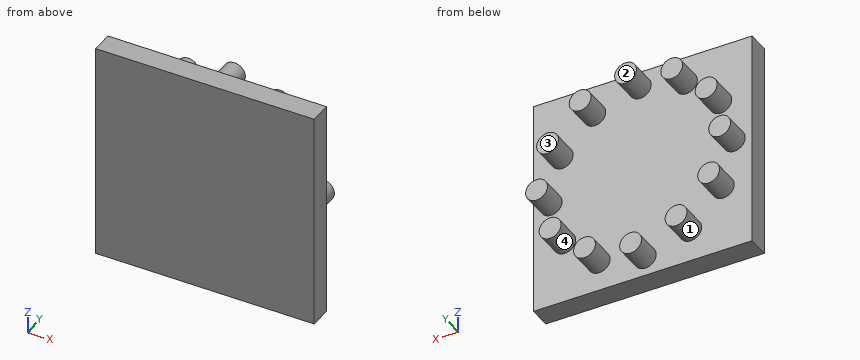
```python
from build123d import *

# Parameters (mm, degrees)
CROQUIS1_W              = 100
CROQUIS1_H              = 100
SALIENTE_EXTRUIR1_DEPTH = 10
CROQUIS2_R              = 5
SALIENTE_EXTRUIR2_DEPTH = 12
MATRIZC1_COUNT          = 12


with BuildPart() as part:
    # Croquis1 → Saliente-Extruir1 (new body)
    with BuildSketch(Plane(origin=(0, 0, 0), x_dir=(1, 0, 0), z_dir=(0, 1, 0))):
        Rectangle(CROQUIS1_W, CROQUIS1_H)
    extrude(amount=SALIENTE_EXTRUIR1_DEPTH)

    # Croquis2 → Saliente-Extruir2 (add)
    with BuildSketch(Plane(origin=(0, 10, 0), x_dir=(1, 0, 0), z_dir=(0, 1, 0))):
        with Locations(Location((-1.140405964, 41.553542307, 0), (0, 0, 270))):
            Circle(CROQUIS2_R)
    saliente_extruir2 = extrude(amount=SALIENTE_EXTRUIR2_DEPTH)

    # MatrizC1: Saliente-Extruir2 ×12 about axis
    matrizc1_axis = Axis((0.00902763, 0, 0.32894428), (0, 1, 0))
    for i in range(1, MATRIZC1_COUNT):
        add(saliente_extruir2.rotate(matrizc1_axis, i * 360 / MATRIZC1_COUNT))


solid = part.part
```
Check sheet for the modelled part. Datum: model origin and axes. Units: mm. Face numbers are marked on the shaded views. A direction names the side the tool comes from. Give positions to 0.01 mm unless a question says otherwise; leave off trailing zeros. Write each loop counter-clockwise with the first axis right and the second up, starting at its lowest first coordinate (ties: lowest second). Pieces come first, ordered by that corner, then holes. Notation, with made-up numbers: (0, 84.5) -> (8, 84.5) arc R21 cw to (8, 94.5) -> close; hole circle Ø1 at (19, 53). An arc over 180 degrees is marked (long way). Use CSV: the item, a comma, the result in double quotes. Start each with the question number.
Q1. Cross-section at D-D on x = -12.5. Enter the section's corners in (y, z), and give its area (3 significant figures).
Q2. Release check for a two-part mould opening along Z. For the marked faces 3 and 4 record: +Z half, -Z half, draft (parallel to the pull), parting line (faces both ways), or undercut.
Q3. Cross-section at A-A on y = 16. Count the separate pieces of the cut face and the enclosed holes in it, and give its area (3 significant figures).
Q4. Depth check by flat-ended pin: P1, Ø6, axis at x = -5, z = 21, coming from the +Y side. Enter the tip coordinate at first touch or a pass-through.
Q5. Cross-section at B-B on x = 39. Enter the section's corners in (y, z), and give its area (3 significant figures).
Q6. Tool access check on the marked faces 1 and 2. Record the directions out of +Z, -Z, +X, -X, +Y, -Y that give a thin tool (end or side, any length) a straight path to the whole face; none if there is none.
Q7. Scan lines: line 1 along Z through (x, y) = (21.5, 11.25); line 2 along Y through (x, z) = (-11.5, -34); line 3 along Z through (x, y) = (42, 19). Record each from-to range of solid material in increasing order.
Q8. Cross-section at C-C on z = 11.5. Enter the section's corners in (x, y).
Working result:
1,outline,"(0, -50) -> (10, -50) -> (10, 50) -> (0, 50) -> close"
1,area,"1,000 mm^2"
2,face 3,"draft"
2,face 4,"undercut"
3,separate pieces,"12"
3,enclosed holes,"0"
3,area,"942 mm^2"
4,P1,"stops at y = 10"
5,outline,"(0, -50) -> (10, -50) -> (10, -25.37) -> (22, -25.37) -> (22, -17.85) -> (10, -17.85) -> (10, -4.9) -> (22, -4.9) -> (22, 3.26) -> (10, 3.26) -> (10, 15.76) -> (22, 15.76) -> (22, 24.79) -> (10, 24.79) -> (10, 50) -> (0, 50) -> close"
5,area,"1,300 mm^2"
6,face 1,"+Y"
6,face 2,"+Z, -Z, +X, -X, +Y"
7,line 1,"z = -41.27 to -31.76, 31.05 to 41.01"
7,line 2,"y = 0 to 10"
7,line 3,"z = -5.82 to 4.18"
8,outline,"(-50, 0) -> (50, 0) -> (50, 10) -> (-50, 10) -> close"
